Could you check a few things on this model? Use its own coordinates, in mm. A direction names the side the tool comes from. Coordinates: 2 decimals unless noted, no trailing zeros. Loops run counter-clockwise (first coordinate to the right, second up) from the corner with the lowest first, then second, coordinate; pieces in that order, holes last. Notation, with made-up numbers: M -19,37 L -5,37 A19 ccw -5,49 Z; hole C 69,-8 d4. An arc over 180 degrees is marked long. Write each question's results on one line, items separated by ' | '.
```python
from build123d import *

# Parameters (mm, degrees)
BOSS_EXTRUDE1_START = -1.675
SKETCH2_R           = 0.5
BOSS_EXTRUDE1_DEPTH = 1.675
CIRPATTERN1_COUNT   = 2
SKETCH3_R           = 0.5
BOSS_EXTRUDE2_DEPTH = 1.675
SKETCH4_R           = 0.5
BOSS_EXTRUDE3_DEPTH = 1.675


with BuildPart() as part:
    # Sketch1 → Revolve1 (revolve)
    with BuildSketch(Plane.XY, mode=Mode.PRIVATE) as revolve1_sk:
        Polygon((2.25, 0), (1.25, 0), (1.25, 0.76), (2, 0.76), (2, 1.69), (3.5, 1.69), (3.5, -2.21), (2.25, -2.21), align=None)
    revolve(revolve1_sk.sketch.rotate(Axis((0, 0, 0), (0, -1, 0)), 180), axis=Axis((0, 0, 0), (0, -1, 0)))

    # Sketch2 → Boss-Extrude1 (add)
    with BuildSketch(Plane(origin=(0, 1.69, 0), x_dir=(1, 0, 0), z_dir=(0, 1, 0)).offset(BOSS_EXTRUDE1_START)):
        with BuildLine():
            Line((-1.905, 6.5278), (-1.905, 2.93614969))
            ThreePointArc((-1.905, 2.93614969), (0, 3.5), (1.905, 2.93614969))
            Line((1.905, 2.93614969), (1.905, 6.5278))
            ThreePointArc((1.905, 6.5278), (0, 8.4328), (-1.905, 6.5278))
        make_face()
        with Locations(Location((0, 6.5278, 0), (0, 0, 180))):
            Circle(SKETCH2_R, mode=Mode.SUBTRACT)
        with Locations(Location((0, 4.5278, 0), (0, 0, 180))):
            Circle(SKETCH2_R, mode=Mode.SUBTRACT)
    boss_extrude1 = extrude(amount=BOSS_EXTRUDE1_DEPTH)

    # CirPattern1: Boss-Extrude1 ×2 about axis
    cirpattern1_axis = Axis((0, 0, 0), (0, 1, 0))
    for i in range(1, CIRPATTERN1_COUNT):
        add(boss_extrude1.rotate(cirpattern1_axis, i * 360 / CIRPATTERN1_COUNT))

    # Sketch3 → Boss-Extrude2 (add)
    with BuildSketch(Plane.XZ.offset(-0.015)):
        with BuildLine():
            Line((0.927024811, -3.375), (16.738893675, -1.929453741))
            ThreePointArc((16.738893675, -1.929453741), (18.5, 0), (16.738893675, 1.929453741))
            Line((16.738893675, 1.929453741), (0.927024811, 3.375))
            ThreePointArc((0.927024811, 3.375), (3.5, 0), (0.927024811, -3.375))
        make_face()
        with Locations((16.562499938, 0)):
            Circle(SKETCH3_R, mode=Mode.SUBTRACT)
        with Locations((14.562499938, 0)):
            Circle(SKETCH3_R, mode=Mode.SUBTRACT)
        with Locations((12.562499938, 0)):
            Circle(SKETCH3_R, mode=Mode.SUBTRACT)
        with Locations((10.562499938, 0)):
            Circle(SKETCH3_R, mode=Mode.SUBTRACT)
        with Locations((8.562499938, 0)):
            Circle(SKETCH3_R, mode=Mode.SUBTRACT)
        with Locations((6.562499938, 0)):
            Circle(SKETCH3_R, mode=Mode.SUBTRACT)
        with Locations((4.562499938, 0)):
            Circle(SKETCH3_R, mode=Mode.SUBTRACT)
    extrude(amount=-BOSS_EXTRUDE2_DEPTH)

    # Sketch4 → Boss-Extrude3 (add)
    with BuildSketch(Plane.XZ.offset(-0.015)):
        with BuildLine():
            Line((-1.905, 2.93614969), (-14.220100787, 1.931079611))
            ThreePointArc((-14.220100787, 1.931079611), (-16, 0), (-14.220100787, -1.931079611))
            Line((-14.220100787, -1.931079611), (-1.905, -2.93614969))
            ThreePointArc((-1.905, -2.93614969), (-3.5, 0), (-1.905, 2.93614969))
        make_face()
        with Locations((-14.062499938, 0)):
            Circle(SKETCH4_R, mode=Mode.SUBTRACT)
        with Locations((-11.562499938, 0)):
            Circle(SKETCH4_R, mode=Mode.SUBTRACT)
        with Locations((-9.062499938, 0)):
            Circle(SKETCH4_R, mode=Mode.SUBTRACT)
        with Locations((-6.562499938, 0)):
            Circle(SKETCH4_R, mode=Mode.SUBTRACT)
        with Locations((-4.062499938, 0)):
            Circle(SKETCH4_R, mode=Mode.SUBTRACT)
    extrude(amount=-BOSS_EXTRUDE3_DEPTH)


solid = part.part
```
(1) Will these pins go through, and if not, where does the flat tip stop? P1, Ø1.2, axis at x = -0.5, z = 1, coming from the +Y side; P2, Ø0.8, axis at y = 0.5, z = -5.5, coming from the +X side (3 decimals); P3, Ø0.8, axis at y = 1, z = 5, coming from the -X side (3 decimals).
Reported:
P1: stops at y = 0.76 | P2: stops at x = 1.905 | P3: stops at x = -1.905
(2) Which directions (+Z, -Z, +X, -X, +Y, -Y) give clear straight access to the entire face, cutting with the end or side of a thin tool? Please do faces 5 (the flat face through (1.905, 1, -5)), 6 (the cylindrical face through (1.66, -1.09, -1.52)), 7 (the flat face through (-1.905, 1, 5)).
Reported:
face 5: -Z, +X, +Y, -Y | face 6: -Y | face 7: +Z, -X, +Y, -Y
(3) Imagine slicing it at B-B, the plane y = -1.75. List the corners of the cut face in (x, z) for me, and give its area (3 significant figures).
Reported:
outline: C 0,0 d7; hole C 0,0 d4.5 | area: 22.6 mm2
(4) If we mould it in two halves opening along X, with no side actions, what happens to faces 1 (the flat face through (-7.98, 0.84, 2.44)), 2 (the flat face through (9.218, 0.841, -2.617)), 3 (the cylindrical face through (0, 1, 2)), 4 (the cylindrical face through (0.042, 0.841, -8.432))? For each: released by +X, released by -X, zero draft, split by the parting line, or undercut.
Reported:
face 1: released by -X | face 2: released by +X | face 3: undercut | face 4: split by the parting line
(5) Imagine slicing it at A-A, the plane x = 0. State how many separate pieces and enclosed holes the cut face has, and give its area (3 significant figures).
Reported:
separate pieces: 6 | enclosed holes: 0 | area: 21.6 mm2
(6) Please list where these lines run through material, in increasing order: probe 1 along X at (y, z) = (0.25, -6.5) (3 decimals); probe 2 along Y at (x, z) = (-0.5, 6.75) (3 decimals); probe 3 along Z at (x, y) = (16, 0.5). Write a range as from..to.
Reported:
probe 1: x = -1.905..-0.499, 0.499..1.905 | probe 2: y = 0.015..1.69 | probe 3: z = -2..2
